Geometry: final body of the model. Coordinates: model frame, mm. Round coordinates to 2 decimals unless told otherwise and drop trailing zeros. Order: outer loops, then holes, each group sorted by start corner. A loop starts at its lowest first (then second) coordinate and runs counter-clockwise, first axis right, second up. Notation, with made-up numbers: (65.25, 23) -> (95.25, 23) arc R13 cw to (95.25, 44) -> close; hole circle Ø8 at (-24, 13). An arc over 180 degrees is marked (long way). Put each result on its own line as item: value.
Autodesk Fusion 360 part; units mm, degrees
sketch "Esboço1" plane through (0, 0, 0) normal (0, 1, 0) x (1, 0, 0)
  line L0 (0, 0) -> (-56, 0)
  line L1 (-56, 0) -> (-56, -20)
  line L2 (-56, -20) -> (0, -20)
  line L3 (0, -20) -> (0, 0)
  dimension "d1" = 56
  dimension "d2" = 20
extrude "Extrusão1" add sketch "Esboço1" along normal blind 13.9
fillet "Arredondamento1" radius 9.9 2 edges at (-28, 13.9, 20) (-28, 13.9, 0)
fillet "Fillet2" radius 2 2 edges at (0, 0, 10) (-56, 0, 10)
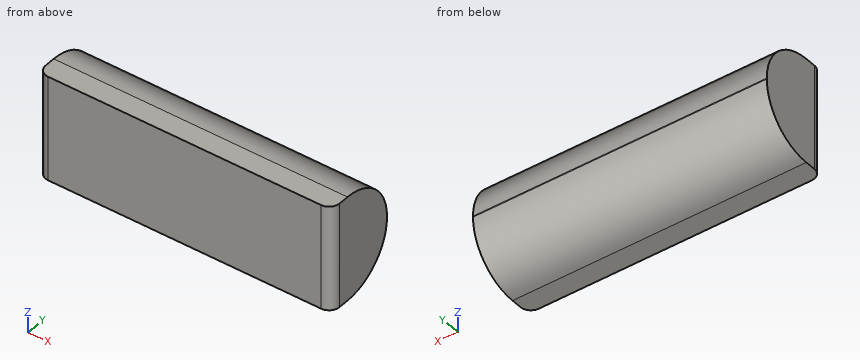
1. Cut plane C-C on y = 12.25. Return loops of the section in (x, z), and give its area (3 significant figures).
Ans:
outline: (-56, 4.43) -> (0, 4.43) -> (0, 15.57) -> (-56, 15.57) -> close
area: 624 mm²
2. Cut plane D-D on y = 7. Return loops of the section in (x, z), and give its area (3 significant figures).
Ans:
outline: (-56, 0.47) -> (0, 0.47) -> (0, 19.53) -> (-56, 19.53) -> close
area: 1,070 mm²
3. Cut plane A-A on x = -17. Return loops of the section in (y, z).
Ans:
outline: (0, 0) -> (4, 0) arc R9.9 ccw to (13.9, 9.9) -> (13.9, 10.1) arc R9.9 ccw to (4, 20) -> (0, 20) -> close
4. Material intervals for probe 1 along Z at (x, y) = (-29, 4.25); probe 2 along Y at (x, z) = (-25.5, 13.5); probe 3 along Z at (x, y) = (-49, 11.25), sorted ascending.
Ans:
probe 1: 0 to 20
probe 2: 0 to 13.3
probe 3: 3.16 to 16.84
5. Contact query for flat-ended pins moving along their axis: P1, Ø2, axis at x = -25.5, y = 7, coming from the -Z side; P2, Ø4, axis at x = -40, y = 6.5, coming from the -Z side; P3, Ø2, axis at x = -25, z = 14.5, coming from the +Y side. Output: stop coordinate, or through.
Ans:
P1: z = 0.2
P2: z = 0.01
P3: y = 13.3
6. Cut plane B-B on z = 12.5. Return loops of the section in (x, y), and give its area (3 significant figures).
Ans:
outline: (-56, 2) arc R2 ccw to (-54, 0) -> (-2, 0) arc R2 ccw to (0, 2) -> (0, 13.6) -> (-56, 13.6) -> close
area: 760 mm²
